For this review, take the finished solid that the model builds, in its own axes (mm). A direction names the side the tool comes from. Round coordinates to 2 decimals unless told otherwise and drop trailing zeros. Write each loop counter-clockwise with the first axis right and the second up, starting at its lowest first coordinate (ties: lowest second). Pieces come first, ordered by that corner, then holes. Notation, with made-up numbers: (68.5, 37) -> (110.5, 37) arc R15 cw to (110.5, 48) -> close; hole circle Ø11 at (-26, -10). An arc over 180 degrees is marked (long way). Write each question's results on one line, items separated by ' | '. Start each with the question number.
Item 1: The part is to be moulded in two halves that separate along Z. For faces 4 (the flat face through (-6.959, 61, -161)), 5 (the flat face through (0, 87, -7)), 6 (the flat face through (0, 87, 0)), 7 (the flat face through (2, 126, -157)), say which applies: +Z half, -Z half, draft (parallel to the pull), parting line (faces both ways), or undercut.
Item 2: To check wall thickness, follow line 1 along Z through (x, y) = (-4, 65); line 2 along Z through (x, y) = (-13, 56); line 3 along Z through (x, y) = (-0.5, 8). State the ranges of each line that lie inside material, in increasing order.
Item 3: Clearance check with flat-ended pins moving along their axes: pin 1 (1 mm diameter, centred on x = -7, y = 13.5, fed in from -Z); pin 2 (6 mm diameter, centred on y = 120, z = -68.5, fed in from -X); pin 3 (4 mm diameter, centred on y = 49.5, z = -162, fed in from +X); pin 4 (4 mm diameter, centred on x = -2, y = 57.5, fed in from +Z). State where each tip first meets the part, or that it passes through.
Item 4: Add section A-A (y = 104). State the section outline as (x, z) points.
Item 5: Add section D-D (y = 45.5). State the section outline as (x, z) points.
Item 6: Add section C-C (z = -25). State the section outline as (x, y) points, plus the area to 3 significant figures.
Item 7: Add section B-B (x = 0). State the section outline as (y, z) points.
Item 8: Tool access review of faces 1 (the flat face through (0, 0, -149)), 2 (the cylindrical face through (0.434, 34.834, -3.451)), 3 (the flat face through (6.959, 60, -161)): name each direction out of +Z, -Z, +X, -X, +Y, -Y from which nothing blocks a thin tool from reaching the whole face with its end or side.
from build123d import *

# Parameters (mm, degrees)
EXTRUDE_1_DEPTH      = 7
SKETCH_3_R           = 7.951035335
EXTRUDE_2_DEPTH      = 150
EXTRUDE_3_DEPTH      = 8
EXTRUDE_4_DEPTH      = 2
EXTRUDE_4_DEPTH_BACK = 16
SKETCH_5_R           = 7.270551731


with BuildPart() as part:
    # 草图1 → 凸台-拉伸1 (new body)
    with BuildSketch(Plane.XY):
        with BuildLine():
            Line((-19.757797481, 54.586532616), (-19.757797481, 118.7433895))
            ThreePointArc((-19.757797481, 118.7433895), (0, 138.50118698), (19.757797481, 118.7433895))
            Line((19.757797481, 118.7433895), (19.757797481, 54.586532616))
            ThreePointArc((19.757797481, 54.586532616), (0, 34.828735136), (-19.757797481, 54.586532616))
        make_face()
    extrude(amount=-EXTRUDE_1_DEPTH)

    # 草图3 → 凸台-拉伸2 (add)
    with BuildSketch(Plane(origin=(0, 0, -7), x_dir=(-1, 0, 0), z_dir=(0, 0, -1))):
        with Locations(Location((0, 118.7433895, 0), (0, 0, 180))):
            Circle(SKETCH_3_R)
    extrude(amount=EXTRUDE_2_DEPTH)

    # 草图4 → 凸台-拉伸3 (add)
    with BuildSketch(Plane(origin=(0, 0, -157), x_dir=(-1, 0, 0), z_dir=(0, 0, -1))):
        with BuildLine():
            Line((6.958683776, 118.7433895), (6.958683776, 0))
            ThreePointArc((6.958683776, 0), (0, -6.958683776), (-6.958683776, 0))
            Line((-6.958683776, 0), (-6.958683776, 118.7433895))
            ThreePointArc((-6.958683776, 118.7433895), (0, 125.702073275), (6.958683776, 118.7433895))
        make_face()
    extrude(amount=EXTRUDE_3_DEPTH)

    # 草图5 → 凸台-拉伸4 (add, two sides: drawn at the far end of the back side and taken through both)
    with BuildSketch(Plane(origin=(0, 0, -165), x_dir=(-1, 0, 0), z_dir=(0, 0, -1)).offset(-EXTRUDE_4_DEPTH_BACK)):
        Circle(SKETCH_5_R)
    extrude(amount=EXTRUDE_4_DEPTH + EXTRUDE_4_DEPTH_BACK)


solid = part.part
Responses:
1) face 4: draft | face 5: undercut | face 6: +Z half | face 7: -Z half
2) line 1: z = -165 to -157, -7 to 0 | line 2: z = -7 to 0 | line 3: z = -165 to -157
3) pin 1: stops at z = -165 | pin 2: stops at x = -7.95 | pin 3: stops at x = 6.96 | pin 4: stops at z = 0
4) outline: (-19.76, -7) -> (19.76, -7) -> (19.76, 0) -> (-19.76, 0) -> close; (-6.96, -165) -> (6.96, -165) -> (6.96, -157) -> (-6.96, -157) -> close
5) outline: (-17.54, -7) -> (17.54, -7) -> (17.54, 0) -> (-17.54, 0) -> close; (-6.96, -165) -> (6.96, -165) -> (6.96, -157) -> (-6.96, -157) -> close
6) outline: circle Ø15.9 at (0, 118.74) | area: 199 mm^2
7) outline: (-7.27, -167) -> (7.27, -167) -> (7.27, -165) -> (125.7, -165) -> (125.7, -157) -> (126.69, -157) -> (126.69, -7) -> (138.5, -7) -> (138.5, 0) -> (34.83, 0) -> (34.83, -7) -> (110.79, -7) -> (110.79, -157) -> (7.27, -157) -> (7.27, -149) -> (-7.27, -149) -> close
8) face 1: +Z, +X, -X, -Y | face 2: +Z, -Y | face 3: -Z, +X, +Y
